Verification items for this drawing (mm, ordinates from the low corner). Round coordinates to 2 decimals unless told otherwise and drop trailing zeros. Order: outer loops, then holes, each group sorted by start corner. A loop starts at its lowest first (then second) coordinate and runs counter-clockwise, first axis right, second up. Notation, with made-up numbers: (-32, -35) - (-24, -35) arc R24 cw to (-24, 0) - close; hole circle Ø2 at (49.5, 25.5). An arc over 180 degrees is marked (long way). One line per question, with ' | ' between items. Start each with the question number.
Q1. Sectioned sample at C-C, the plane x = 5.75. Enter the section's corners in (y, z).
Q2. Sectioned sample at B-B, the plane y = 4.75. Enter the section's corners in (x, z).
Q3. Material ranges on line 1 along Y through (x, z) = (22, 0.45); line 2 along X through (y, z) = (5.5, 0.7), recorded low to high.
Q4. Sectioned sample at A-A, the plane z = 0.3. Enter the section's corners in (x, y).
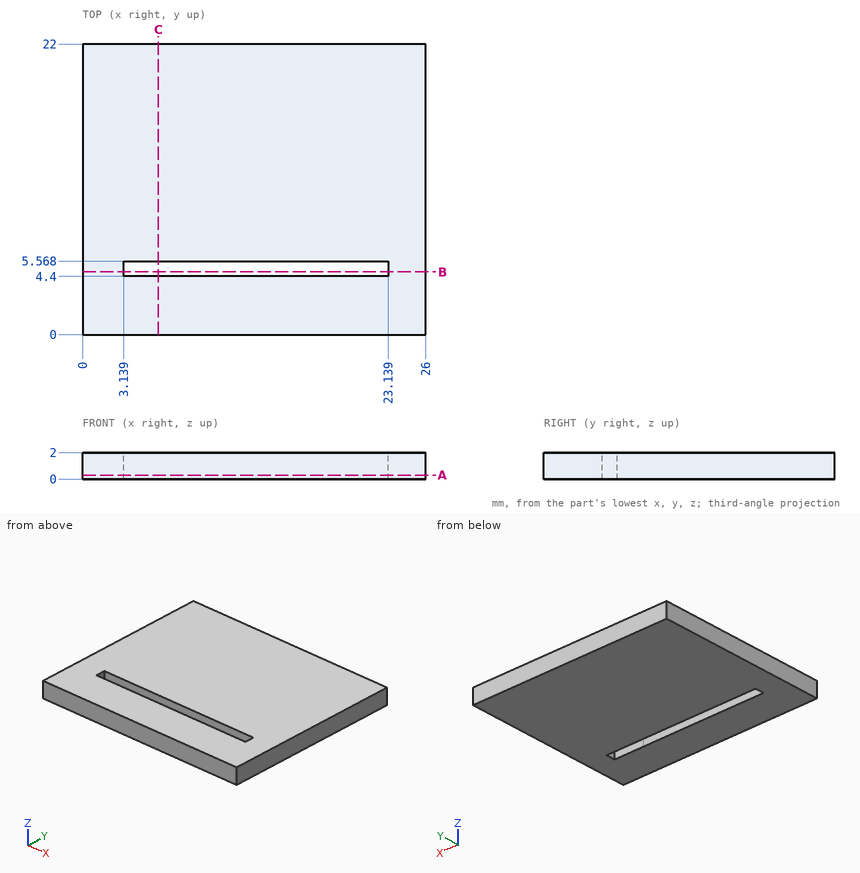
Determined:
1) outline: (0, 0) - (4.4, 0) - (4.4, 2) - (0, 2) - close; (5.57, 0) - (22, 0) - (22, 2) - (5.57, 2) - close
2) outline: (0, 0) - (3.14, 0) - (3.14, 2) - (0, 2) - close; (23.14, 0) - (26, 0) - (26, 2) - (23.14, 2) - close
3) line 1: y = 0 to 4.4, 5.57 to 22 | line 2: x = 0 to 3.14, 23.14 to 26
4) outline: (0, 0) - (26, 0) - (26, 22) - (0, 22) - close; hole (3.14, 4.4) - (23.14, 4.4) - (23.14, 5.57) - (3.14, 5.57) - close
